Model file for the job. Use its own axes, mm. A direction names the side the tool comes from. Coordinates: 2 decimals unless noted, no trailing zeros. Order: outer loops, then holes, each group sorted by start corner. A loop starts at its lowest first (then second) coordinate and runs counter-clockwise, first axis right, second up. Notation, with made-up numbers: (74.5, -18.5) -> (81.5, -18.5) arc R30 ccw to (81.5, 8.5) -> close; hole circle Ø3 at (-3.75, 56.25). An arc over 180 degrees is marked (long way). Return JSON: item names as keys, results as strings. Group by question number.
1) Cut at B-B (x = 5). Write the cut outline in (y, z).
2) Cut at A-A (y = -1). State how many separate pieces and enclosed holes the cut face has, and give its area (3 significant figures).
3) Which spindle directions (+Z, -Z, +X, -X, +Y, -Y) get a long thin tool onto all of the face, cutting with end or side? Do faces 4 (the cylindrical face through (6.386, -2.465, 0.575)), 5 (the flat face through (-3, 2, 2)), 6 (the cylindrical face through (-1.694, 1.493, 1.235)). Say none if no direction does.
4) Flat gauge pins, fed straight in: pin 1 (2.5 mm diameter, centred on x = -5.5, z = -0.5, fed in from -Y); pin 2 (3 mm diameter, centred on x = -5, z = -0.5, fed in from +Y); pin 3 (1.8 mm diameter, centred on x = -5, z = 0, fed in from -Y). Where does each tip first touch, or does it go through?
5) Pull direction X, two halves, no side cores. Call faces 1 (the flat face through (-15, -2, 0)), 2 (the flat face through (14, -2, 0)), 3 (the flat face through (-8, 2, 2)): +X half, -X half, draft (parallel to the pull), parting line (faces both ways), or undercut.
6) Probe line 1 (Z direction, x = 10, y = -1.4); line 2 (Z direction, x = -12.75, y = -4.25); line 3 (X direction, y = -2, z = -2.5). List the from-to ranges inside material, lowest first.
from build123d import *

# Parameters (mm, degrees)
SKETCH1_R              = 1.5
BOSS_EXTRUDE1_DEPTH    = 2
BOSS_EXTRUDE1_2_DEPTH  = 2
BOSS_EXTRUDE1_3_DEPTH  = 2
BOSS_EXTRUDE1_4_DEPTH  = 2
BOSS_EXTRUDE1_5_DEPTH  = 2
BOSS_EXTRUDE1_6_DEPTH  = 2
BOSS_EXTRUDE1_7_DEPTH  = 2
BOSS_EXTRUDE1_8_DEPTH  = 2
BOSS_EXTRUDE1_9_DEPTH  = 2
BOSS_EXTRUDE1_10_DEPTH = 2
BOSS_EXTRUDE1_11_DEPTH = 2
BOSS_EXTRUDE1_12_DEPTH = 2
SKETCH1_3_W            = 30
SKETCH1_3_H            = 10
BOSS_EXTRUDE2_DEPTH    = 1
SKETCH1_4_W            = 30
SKETCH1_4_H            = 10
SKETCH1_4_W_2          = 28
SKETCH1_4_H_2          = 8
SKETCH1_4_R            = 2.035533906
SKETCH1_4_R_2          = 1.5
BOSS_EXTRUDE3_DEPTH    = 5


with BuildPart() as part:
    # Sketch1 → Boss-Extrude1 (new body)
    with BuildSketch(Plane(origin=(0, 0, 0), x_dir=(1, 0, 0), z_dir=(0, 1, 0))):
        with Locations((-2.5, 2.5)):
            Circle(SKETCH1_R)
    extrude(amount=BOSS_EXTRUDE1_DEPTH)



with BuildPart() as body_2:
    # Sketch1 → Boss-Extrude1 2 (new body)
    with BuildSketch(Plane(origin=(0, 0, 0), x_dir=(1, 0, 0), z_dir=(0, 1, 0))):
        with Locations((-7.5, 2.5)):
            Circle(SKETCH1_R)
    extrude(amount=BOSS_EXTRUDE1_2_DEPTH)


with BuildPart() as body_3:
    # Sketch1 → Boss-Extrude1 3 (new body)
    with BuildSketch(Plane(origin=(0, 0, 0), x_dir=(1, 0, 0), z_dir=(0, 1, 0))):
        with Locations((-12.5, 2.5)):
            Circle(SKETCH1_R)
    extrude(amount=BOSS_EXTRUDE1_3_DEPTH)


with BuildPart() as body_4:
    # Sketch1 → Boss-Extrude1 4 (new body)
    with BuildSketch(Plane(origin=(0, 0, 0), x_dir=(1, 0, 0), z_dir=(0, 1, 0))):
        with Locations((-12.5, -2.5)):
            Circle(SKETCH1_R)
    extrude(amount=BOSS_EXTRUDE1_4_DEPTH)


with BuildPart() as body_5:
    # Sketch1 → Boss-Extrude1 5 (new body)
    with BuildSketch(Plane(origin=(0, 0, 0), x_dir=(1, 0, 0), z_dir=(0, 1, 0))):
        with Locations((-7.5, -2.5)):
            Circle(SKETCH1_R)
    extrude(amount=BOSS_EXTRUDE1_5_DEPTH)


with BuildPart() as body_6:
    # Sketch1 → Boss-Extrude1 6 (new body)
    with BuildSketch(Plane(origin=(0, 0, 0), x_dir=(1, 0, 0), z_dir=(0, 1, 0))):
        with Locations((-2.5, -2.5)):
            Circle(SKETCH1_R)
    extrude(amount=BOSS_EXTRUDE1_6_DEPTH)


with BuildPart() as body_7:
    # Sketch1 → Boss-Extrude1 7 (new body)
    with BuildSketch(Plane(origin=(0, 0, 0), x_dir=(1, 0, 0), z_dir=(0, 1, 0))):
        with Locations((2.5, 2.5)):
            Circle(SKETCH1_R)
    extrude(amount=BOSS_EXTRUDE1_7_DEPTH)


with BuildPart() as body_8:
    # Sketch1 → Boss-Extrude1 8 (new body)
    with BuildSketch(Plane(origin=(0, 0, 0), x_dir=(1, 0, 0), z_dir=(0, 1, 0))):
        with Locations((7.5, 2.5)):
            Circle(SKETCH1_R)
    extrude(amount=BOSS_EXTRUDE1_8_DEPTH)


with BuildPart() as body_9:
    # Sketch1 → Boss-Extrude1 9 (new body)
    with BuildSketch(Plane(origin=(0, 0, 0), x_dir=(1, 0, 0), z_dir=(0, 1, 0))):
        with Locations((12.5, 2.5)):
            Circle(SKETCH1_R)
    extrude(amount=BOSS_EXTRUDE1_9_DEPTH)


with BuildPart() as body_10:
    # Sketch1 → Boss-Extrude1 10 (new body)
    with BuildSketch(Plane(origin=(0, 0, 0), x_dir=(1, 0, 0), z_dir=(0, 1, 0))):
        with Locations((12.5, -2.5)):
            Circle(SKETCH1_R)
    extrude(amount=BOSS_EXTRUDE1_10_DEPTH)


with BuildPart() as body_11:
    # Sketch1 → Boss-Extrude1 11 (new body)
    with BuildSketch(Plane(origin=(0, 0, 0), x_dir=(1, 0, 0), z_dir=(0, 1, 0))):
        with Locations((7.5, -2.5)):
            Circle(SKETCH1_R)
    extrude(amount=BOSS_EXTRUDE1_11_DEPTH)


with BuildPart() as body_12:
    # Sketch1 → Boss-Extrude1 12 (new body)
    with BuildSketch(Plane(origin=(0, 0, 0), x_dir=(1, 0, 0), z_dir=(0, 1, 0))):
        with Locations((2.5, -2.5)):
            Circle(SKETCH1_R)
    extrude(amount=BOSS_EXTRUDE1_12_DEPTH)


with BuildPart() as part_1:
    add(part.part)

    add(body_2.part)  # Boss-Extrude2 merges body 2

    add(body_3.part)  # Boss-Extrude2 merges body 3

    add(body_4.part)  # Boss-Extrude2 merges body 4

    add(body_5.part)  # Boss-Extrude2 merges body 5

    add(body_6.part)  # Boss-Extrude2 merges body 6

    add(body_7.part)  # Boss-Extrude2 merges body 7

    add(body_8.part)  # Boss-Extrude2 merges body 8

    add(body_9.part)  # Boss-Extrude2 merges body 9

    add(body_10.part)  # Boss-Extrude2 merges body 10

    add(body_11.part)  # Boss-Extrude2 merges body 11

    add(body_12.part)  # Boss-Extrude2 merges body 12
    # Sketch1_3 → Boss-Extrude2 (add)
    with BuildSketch(Plane(origin=(0, 0, 0), x_dir=(1, 0, 0), z_dir=(0, 1, 0))):
        Rectangle(SKETCH1_3_W, SKETCH1_3_H)
    extrude(amount=BOSS_EXTRUDE2_DEPTH)

    # Sketch1_4 → Boss-Extrude3 (add)
    with BuildSketch(Plane(origin=(0, 0, 0), x_dir=(1, 0, 0), z_dir=(0, 1, 0))):
        Rectangle(SKETCH1_4_W, SKETCH1_4_H)
        Rectangle(SKETCH1_4_W_2, SKETCH1_4_H_2, mode=Mode.SUBTRACT)
        with Locations((-10, 0)):
            Circle(SKETCH1_4_R)
        with Locations((-10, 0)):
            Circle(SKETCH1_4_R_2, mode=Mode.SUBTRACT)
        with Locations((-5, 0)):
            Circle(SKETCH1_4_R)
        with Locations((-5, 0)):
            Circle(SKETCH1_4_R_2, mode=Mode.SUBTRACT)
        Circle(SKETCH1_4_R)
        Circle(SKETCH1_4_R_2, mode=Mode.SUBTRACT)
        with Locations((5, 0)):
            Circle(SKETCH1_4_R)
        with Locations((5, 0)):
            Circle(SKETCH1_4_R_2, mode=Mode.SUBTRACT)
        with Locations((10, 0)):
            Circle(SKETCH1_4_R)
        with Locations((10, 0)):
            Circle(SKETCH1_4_R_2, mode=Mode.SUBTRACT)
    extrude(amount=-BOSS_EXTRUDE3_DEPTH)


solid = part_1.part
Answers below:
{
 "1": {"outline": "(-5, -5) -> (1, -5) -> (1, 5) -> (-5, 5) -> (-5, 4) -> (0, 4) -> (0, 2.04) -> (-5, 2.04) -> (-5, 1.5) -> (0, 1.5) -> (0, -1.5) -> (-5, -1.5) -> (-5, -2.04) -> (0, -2.04) -> (0, -4) -> (-5, -4) -> close"},
 "2": {"separate pieces": "6", "enclosed holes": "6", "area": "106 mm^2"},
 "3": {"face 4": "-Y", "face 5": "+Z, -Z, +X, -X, +Y", "face 6": "+Y"},
 "4": {"pin 1": "stops at y = -5", "pin 2": "stops at y = 1", "pin 3": "stops at y = 0"},
 "5": {"face 1": "-X half", "face 2": "undercut", "face 3": "draft"},
 "6": {"line 1": "z = -5 to -4, -2.04 to -1.5, 1.5 to 2.04, 4 to 5", "line 2": "z = -5 to -4, 4 to 5", "line 3": "x = -15 to -14, 14 to 15"}
}
